The listing builds one solid part. Answer for the finished solid, in the listing's coordinates (mm). A direction names the side the tool comes from. Coordinates: 2 decimals unless noted, no trailing zeros. Write each loop counter-clockwise with the first axis right and the second up, starting at its lowest first coordinate (ties: lowest second). Pieces come first, ordered by that corner, then holes.
from build123d import *

# Parameters (mm, degrees)
F0_R     = 45
F1_DEPTH = 200
F1_TAPER = -10
F2_R     = 75
F3_DEPTH = 195
F3_TAPER = 10
F5_W     = 13.1450463086
F5_H     = 17.6969505847
F6_DEPTH = 268


with BuildPart() as f1:
    # F0 (on Top) → F1 (new body)
    with BuildSketch(Plane.XY):
        Circle(F0_R)
    extrude(amount=F1_DEPTH, taper=F1_TAPER)

    # F2 (on face) → F3 (cut)
    with BuildSketch(Plane.XY.offset(200)):
        Circle(F2_R)
    extrude(amount=-F3_DEPTH, taper=F3_TAPER, mode=Mode.SUBTRACT)

    # F5 (on offset) → F6 (join)
    with BuildSketch(Plane.XY.offset(5)):
        with Locations((-6.5725231543, 8.8484752923)):
            Rectangle(F5_W, F5_H)
    extrude(amount=F6_DEPTH)


solid = f1.part
1. A tool of negligible diameter and unlimited length cuts with its end or side. For faces 4 (the flat face through (-1, 1, 0)), 5 (the flat face through (0, 9, 137)), from which of +Z, -Z, +X, -X, +Y, -Y can it reach the whole face along a straight path? Write none if from no direction.
Results found:
face 4: -Z, +X, -X, +Y, -Y
face 5: +Z
2. Flat-ended cylindrical pins translate along their axes: P1, Ø10.5, axis at x = -6, z = 145, coming from the +Y side; P2, Ø3, axis at x = 19, z = 74.5, coming from the +Y side; P3, Ø10.5, axis at x = -5.5, z = 139, coming from the -Y side. Find the tip coordinate at first contact, or state that the pin passes through.
Results found:
P1: stops at y = 71.31
P2: stops at y = 55.51
P3: stops at y = -70.28
3. For a pull along Y with two mould halves and no side action, classify faces 1 (the conical face through (54.9, 17.3, 101.1)), 2 (the conical face through (-13.631, -61.384, 101.4)), 3 (the flat face through (-7, 9, 273)) as pulls with the +Y half, pulls with the -Y half, needs draft (parallel to the pull), parting line crosses it, or undercut.
Results found:
face 1: undercut
face 2: parting line crosses it
face 3: needs draft
4. Section A-A on z = 138.5 is taken. Give the vertices of the cut face in (x, y), then the cut area to 3 significant figures.
Results found:
outline: circle Ø138.84 at (0, 0); (-13.15, 0) - (0, 0) - (0, 17.7) - (-13.15, 17.7) - close; hole circle Ø128.31 at (0, 0)
area: 2,440 mm2
5. Section B-B on z = 42.5 is taken. Give the vertices of the cut face in (x, y).
Results found:
outline: circle Ø104.99 at (0, 0); (-13.15, 0) - (0, 0) - (0, 17.7) - (-13.15, 17.7) - close; hole circle Ø94.46 at (0, 0)
6. Find the intervals of material crossed by L1, parallel to Y at x = -4, z = 149.5; L2, parallel to X at y = 5.5, z = 33.5; L3, parallel to X at y = 9, z = 182, in increasing order.
Results found:
L1: y = -71.25 to -65.97, 0 to 17.7, 65.97 to 71.25
L2: x = -50.61 to -45.31, -13.15 to 0, 45.31 to 50.61
L3: x = -76.56 to -71.26, -13.15 to 0, 71.26 to 76.56
